from build123d import *

# Parameters (mm, degrees)
BOSS_EXTRU_1_DEPTH             = 4
ENL_V_START                    = -4
ENL_V_MAT_EXTRU_3_DEPTH        = 3.6
CONG_2_R                       = 3
CONG_3_R                       = 3
CONG_2_OF_SYM_TRIE1_R          = 3
CONG_3_OF_SYM_TRIE1_R          = 3
F_4_8_4_8_DIAMETER_HOLE2_D     = 4.8
F_4_8_4_8_DIAMETER_HOLE2_DEPTH = 6.4
F_4_8_4_8_DIAMETER_HOLE2_TIP   = 1.442065486
CHANFREIN1_SIZE                = 0.5
ESQUISSE9_R                    = 4.5
ENL_V_MAT_EXTRU_4_DEPTH        = 1.1
CONG_4_R                       = 1
CHANFREIN2_SIZE                = 0.75


with BuildPart() as part:
    # Esquisse1 → Révolution1 (revolve)
    with BuildSketch(Plane.XY, mode=Mode.PRIVATE) as r_volution1_sk:
        Polygon((-6.5, -4), (-6.5, -5.5), (-10, -5.5), (-10, 2.1), (-8, 2.1), (-8, -4), align=None)
    revolve(r_volution1_sk.sketch.rotate(Axis((0, 6.608552154, 0), (0, -1, 0)), 270), axis=Axis((0, 6.608552154, 0), (0, -1, 0)))

    # Esquisse2 → Boss.-Extru.1 (add)
    with BuildSketch(Plane(origin=(0, 2.1, 0), x_dir=(1, 0, 0), z_dir=(0, 1, 0))):
        with BuildLine():
            Line((-12.5, -4), (-9.16515139, -4))
            ThreePointArc((-9.16515139, -4), (-10, 0), (-9.16515139, 4))
            Line((-9.16515139, 4), (-12.5, 4))
            ThreePointArc((-12.5, 4), (-16.5, 0), (-12.5, -4))
        make_face()
    boss_extru_1 = extrude(amount=-BOSS_EXTRU_1_DEPTH)

    # Esquisse2<6> → Enlèv. mat.-Extru.3 (cut)
    with BuildSketch(Plane(origin=(0, 2.1, 0), x_dir=(1, 0, 0), z_dir=(0, 1, 0)).offset(ENL_V_START)):
        with BuildLine():
            ThreePointArc((-9.5, 3.122498999), (-10, 0), (-9.5, -3.122498999))
            Line((-9.5, -3.122498999), (-9.5, 3.122498999))
        make_face()
    enl_v_mat_extru_3 = extrude(amount=-ENL_V_MAT_EXTRU_3_DEPTH, mode=Mode.SUBTRACT)

    # Congé2
    cong_2_edges = [part.edges().sort_by_distance(p)[0] for p in [
        (-9.5, -3.7, 3.122498999),
        (-9.5, -3.7, -3.122498999),
    ]]
    fillet(cong_2_edges, radius=CONG_2_R)

    # Congé3
    cong_3_edges = [part.edges().sort_by_distance(p)[0] for p in [
        (-9.16515139, 0.1, -4),
        (-9.16515139, 0.1, 4),
    ]]
    fillet(cong_3_edges, radius=CONG_3_R)

    # Symétrie1: Boss.-Extru.1, Enlèv. mat.-Extru.3 across plane
    add(boss_extru_1.mirror(Plane(origin=(0, 0, 0), x_dir=(0, 0, 1), z_dir=(1, 0, 0))))
    add(enl_v_mat_extru_3.mirror(Plane(origin=(0, 0, 0), x_dir=(0, 0, 1), z_dir=(1, 0, 0))), mode=Mode.SUBTRACT)

    # Congé2 of Symétrie1
    cong_2_of_sym_trie1_edges = [part.edges().sort_by_distance(p)[0] for p in [
        (9.5, -3.7, 3.122498999),
        (9.5, -3.7, -3.122498999),
    ]]
    fillet(cong_2_of_sym_trie1_edges, radius=CONG_2_OF_SYM_TRIE1_R)

    # Congé3 of Symétrie1
    cong_3_of_sym_trie1_edges = [part.edges().sort_by_distance(p)[0] for p in [
        (9.16515139, 0.1, -4),
        (9.16515139, 0.1, 4),
    ]]
    fillet(cong_3_of_sym_trie1_edges, radius=CONG_3_OF_SYM_TRIE1_R)

    # Ø4.8 (4.8) Diameter Hole2
    with Locations(Plane(origin=(0, 2.1, 0), x_dir=(1, 0, 0), z_dir=(0, 1, 0))):
        with Locations((-12.5, 0), (12.5, 0)):
            Hole(F_4_8_4_8_DIAMETER_HOLE2_D / 2, depth=F_4_8_4_8_DIAMETER_HOLE2_DEPTH)
            with Locations((0, 0, -(F_4_8_4_8_DIAMETER_HOLE2_DEPTH + F_4_8_4_8_DIAMETER_HOLE2_TIP / 2))):  # 118° drill point
                Cone(0, F_4_8_4_8_DIAMETER_HOLE2_D / 2, F_4_8_4_8_DIAMETER_HOLE2_TIP, mode=Mode.SUBTRACT)

    # Chanfrein1
    chanfrein1_edges = [part.edges().sort_by_distance(p)[0] for p in [
        (14.9, 2.1, 0),
        (-10.1, 2.1, 0),
    ]]
    chamfer(chanfrein1_edges, length=CHANFREIN1_SIZE)

    # Esquisse9 → Enlèv. mat.-Extru.4 (cut)
    with BuildSketch(Plane.XZ.offset(5.5)):
        with Locations((-12.5, 0)):
            Circle(ESQUISSE9_R)
        with Locations((12.5, 0)):
            Circle(ESQUISSE9_R)
    extrude(amount=-ENL_V_MAT_EXTRU_4_DEPTH, mode=Mode.SUBTRACT)

    # Congé4
    # the kernel refuses this fillet: 1 mm, written as the material it takes off along each edge
    with BuildSketch(Plane(origin=(9.421052632, -4.4, 3.281780477), x_dir=(-0.686560042836171, 0, -0.7270731102033653), z_dir=(0, -1, 0))) as cong_4_piece_1:
        with BuildLine():
            CenterArc((0.604915781, -0.998168708), CONG_4_R, 93.468029374, 62.964308211)
            Line((-0.311672758, -0.598336932), (-0.403331612, -0.558353754))
            ThreePointArc((-0.403331612, -0.558353754), (-0.310284429, -0.351422835), (-0.083419367, 0.05514716))
            Line((-0.083419367, 0.05514716), (0.006049158, 0.099816871))
            ThreePointArc((0.006049158, 0.099816871), (0.272212102, 0.091759185), (0.538375045, 0.099816871))
            Line((0.538375045, 0.099816871), (0.544424203, 0))
        make_face()
    extrude(amount=2.786614567, mode=Mode.SUBTRACT)
    with BuildSketch(Plane(origin=(9.421052632, -4.4, -3.281780477), x_dir=(-0.6865600428361709, 0, 0.7270731102033654), z_dir=(0, -1, 0)), Plane(origin=(-9.421052632, -4.4, 3.281780477), x_dir=(0.6865600428361707, 0, -0.7270731102033658), z_dir=(0, -1, 0))) as cong_4_piece_2:
        with BuildLine():
            CenterArc((0.604915781, 0.998168708), CONG_4_R, 203.567662416, 62.964308211)
            Line((-0.311672758, 0.598336932), (-0.403331612, 0.558353754))
            ThreePointArc((-0.403331612, 0.558353754), (-0.310284429, 0.351422835), (-0.083419367, -0.05514716))
            Line((-0.083419367, -0.05514716), (0.006049158, -0.099816871))
            ThreePointArc((0.006049158, -0.099816871), (0.272212102, -0.091759185), (0.538375045, -0.099816871))
            Line((0.538375045, -0.099816871), (0.544424203, 0))
        make_face()
    extrude(amount=2.786614567, mode=Mode.SUBTRACT)
    with BuildSketch(Plane(origin=(-9.421052632, -4.4, -3.281780477), x_dir=(0.3276573021844398, 0, -0.9447966407249841), z_dir=(0, -1, 0))) as cong_4_piece_3:
        with BuildLine():
            CenterArc((0.605807396, 0.997627822), CONG_4_R, 210.982965052, 62.964308211)
            Line((-0.251512996, 0.482844619), (-0.337245035, 0.431366299))
            ThreePointArc((-0.337245035, 0.431366299), (-0.207136841, 0.199031418), (-0.091321217, -0.04074844))
            Line((-0.091321217, -0.04074844), (-0.010371424, -0.099460714))
            ThreePointArc((-0.010371424, -0.099460714), (0.455018696, -0.112838034), (0.68152967, -0.099762782))
            Line((0.68152967, -0.099762782), (0.674645827, 0))
        make_face()
    extrude(amount=2.786614567, mode=Mode.SUBTRACT)

    # Chanfrein2
    chanfrein2_edges = [part.edges().sort_by_distance(p)[0] for p in [
        (0, 2.1, -8),
    ]]
    chamfer(chanfrein2_edges, length=CHANFREIN2_SIZE)


solid = part.part
Model file for the job. Use its own axes, mm. A direction names the side the tool comes from. Give positions to 0.01 mm unless a question says otherwise; leave off trailing zeros. Order: outer loops, then holes, each group sorted by start corner. A loop starts at its lowest first (then second) coordinate and runs counter-clockwise, first axis right, second up. Notation, with made-up numbers: M 1,-32.5 L 17,-32.5 A30 cw 17,-9.5 Z; hole C 1.25,62.25 d1. An arc over 180 degrees is marked long. Put each result on its own line as item: value. Start each with the question number.
(1) Band-saw the part on A-A on z = 0. Count the separate pieces of the cut face and the enclosed holes in it, then the cut area to 3 significant figures.
(2) Drill centre lines: L1, parallel to X at y = 0.65, z = 0; L2, parallel to X at y = -0.75, z = -1.5; L3, parallel to X at y = -4.7, z = 0. Where is each one in solid material? Low to high. Write a range as [from, to].
(3) Tool access for faces 5 (the face through (-9.444, -3.168, 3.173)), 6 (the face through (9.444, -3.168, -3.173)), 7 (the face through (-12, 0, 4)), 8 (the face through (9, -4.4, 0)), 9 (the face through (9.5, -3, 0)): list every direction of +Z, -Z, +X, -X, +Y, -Y with a clear straight run to the whole face (end or side of a thin tool).
(4) Pin check, flat tips, straight feed: pin 1 Ø1 at (x, z) = (-9, 6.5) entering from -Y; pin 2 Ø0.8 at (x, z) = (-9, -0.5) entering from -Y; pin 3 Ø0.8 at (x, y) = (11.5, -0.5) entering from -Z; pin 4 Ø2 at (x, y) = (-11, -2) entering from -Z. Stop position of each tip, or through.
(5) Band-saw the part on C-C on y = -3. Give the cut face in (x, z).
(6) Pull direction Z, two halves, no side cores. Call faces 1 (the face through (3.955, -4.76, -5.158)), 2 (the face through (12, 0, 4)), 3 (the face through (-9, -4.4, 0)), 4 (the face through (-9.5, -3, 0)): released by +Z, released by -Z, zero draft, split by the parting line, or undercut.
(7) Band-saw the part on B-B on x = 0. Give the cut face in (y, z), then the cut area to 3 significant figures.
Results below:
1. separate pieces: 4
1. enclosed holes: 0
1. area: 40.5 mm2
2. L1: x = [-16.5, -14.9], [-10.1, -8], [8, 10.1], [14.9, 16.5]
2. L2: x = [-16.21, -14.37], [-10.63, -7.86], [7.86, 10.63], [14.37, 16.21]
2. L3: x = [-8, -6.5], [6.5, 8]
3. face 5: +Z, -X, -Y
3. face 6: -Z, +X, -Y
3. face 7: +Z, -X, +Y, -Y
3. face 8: +X, -Y
3. face 9: +Z, -Z, +X, -Y
4. pin 1: passes through
4. pin 2: stops at y = -4.4
4. pin 3: stops at z = -4
4. pin 4: stops at z = -4.15
5. outline: M -9.5,-2.6 A3 ccw -9.29,-3.71 A10 ccw 9.29,-3.71 A3 ccw 9.5,-2.6 L 9.5,2.6 A3 ccw 9.29,3.71 A10 ccw -9.29,3.71 A3 ccw -9.5,2.6 Z; hole C 0,0 d16
6. face 1: undercut
6. face 2: released by +Z
6. face 3: undercut
6. face 4: zero draft
7. outline: M -5.5,-10 L 2.1,-10 L 2.1,-8.75 L 1.35,-8 L -4,-8 L -4,-6.5 L -5.5,-6.5 Z; M -5.5,6.5 L -4,6.5 L -4,8 L 1.35,8 L 2.1,8.75 L 2.1,10 L -5.5,10 Z
7. area: 34.3 mm2
